```python
from build123d import *

# Parameters (mm, degrees)
SKETCH1_R               = 15
SKETCH1_R_2             = 1.55
BOSS_EXTRUDE1_DEPTH     = 2.8
BOSS_EXTRUDE2_START     = 2.8
SKETCH3_R               = 7.6
BOSS_EXTRUDE2_DEPTH     = 11
CUT_EXTRUDE1_DEPTH      = 26.306916051
CUT_EXTRUDE1_DEPTH_BACK = 26.306916051
SKETCH4_R               = 2.5
SKETCH5_R               = 5
CUT_EXTRUDE2_DEPTH      = 5.5
BOSS_EXTRUDE3_START     = 12
SKETCH7_R               = 7.6
SKETCH7_R_2             = 3.2
BOSS_EXTRUDE3_DEPTH     = 12
SKETCH8_R               = 3.2
SKETCH8_R_2             = 2.5
BOSS_EXTRUDE4_DEPTH     = 8
BOSS_EXTRUDE5_START     = 3
SKETCH9_R               = 8.25
SKETCH9_R_2             = 7.6
BOSS_EXTRUDE5_DEPTH     = 3
FILLET2_R               = 1
BOSS_EXTRUDE6_START     = 5.5
SKETCH11_R              = 5
SKETCH11_R_2            = 2.5
BOSS_EXTRUDE6_DEPTH     = 5.5
CUT_EXTRUDE3_DEPTH      = 5.5
BOSS_EXTRUDE7_START     = -18.3
SKETCH12_R              = 2.5
BOSS_EXTRUDE7_DEPTH     = 13.3


with BuildPart() as part:
    # Sketch1 → Boss-Extrude1 (new body)
    with BuildSketch(Plane.XY):
        Circle(SKETCH1_R)
        with Locations((0, 12.5)):
            Circle(SKETCH1_R_2, mode=Mode.SUBTRACT)
        with Locations((12.5, 0)):
            Circle(SKETCH1_R_2, mode=Mode.SUBTRACT)
        with Locations((0, -12.5)):
            Circle(SKETCH1_R_2, mode=Mode.SUBTRACT)
        with Locations((-12.5, 0)):
            Circle(SKETCH1_R_2, mode=Mode.SUBTRACT)
    extrude(amount=BOSS_EXTRUDE1_DEPTH)

    # Sketch3 → Boss-Extrude2 (add)
    with BuildSketch(Plane.XY.offset(BOSS_EXTRUDE2_START)):
        Circle(SKETCH3_R)
    extrude(amount=BOSS_EXTRUDE2_DEPTH)

    # Sketch4 → Cut-Extrude1 (cut, two sides: drawn at the far end of the back side and taken through both)
    with BuildSketch(Plane.XY.offset(13.8).offset(-CUT_EXTRUDE1_DEPTH_BACK)):
        Circle(SKETCH4_R)
    extrude(amount=CUT_EXTRUDE1_DEPTH + CUT_EXTRUDE1_DEPTH_BACK, mode=Mode.SUBTRACT)

    # Sketch5 → Cut-Extrude2 (cut)
    with BuildSketch(Plane.XY.offset(13.8)):
        Circle(SKETCH5_R)
    extrude(amount=-CUT_EXTRUDE2_DEPTH, mode=Mode.SUBTRACT)

    # Sketch7 → Boss-Extrude3 (add)
    with BuildSketch(Plane(origin=(0, 0, 0), x_dir=(-1, 0, 0), z_dir=(0, 0, -1)).offset(BOSS_EXTRUDE3_START)):
        with Locations(Location((0, 0, 0), (0, 0, 180))):
            Circle(SKETCH7_R)
        Circle(SKETCH7_R_2, mode=Mode.SUBTRACT)
    extrude(amount=-BOSS_EXTRUDE3_DEPTH)

    # Sketch8 → Boss-Extrude4 (add)
    with BuildSketch(Plane(origin=(0, 0, 0), x_dir=(-1, 0, 0), z_dir=(0, 0, -1))):
        Circle(SKETCH8_R)
        with Locations(Location((0, 0, 0), (0, 0, 180))):
            Circle(SKETCH8_R_2, mode=Mode.SUBTRACT)
    extrude(amount=BOSS_EXTRUDE4_DEPTH)

    # Sketch9 → Boss-Extrude5 (add)
    with BuildSketch(Plane(origin=(0, 0, 0), x_dir=(-1, 0, 0), z_dir=(0, 0, -1)).offset(BOSS_EXTRUDE5_START)):
        with Locations(Location((0, 0, 0), (0, 0, 180))):
            Circle(SKETCH9_R)
        with Locations(Location((0, 0, 0), (0, 0, 180))):
            Circle(SKETCH9_R_2, mode=Mode.SUBTRACT)
    extrude(amount=-BOSS_EXTRUDE5_DEPTH)

    # Fillet2
    fillet2_edges = [part.edges().sort_by_distance(p)[0] for p in [
        (-8.25, 0, 0),
    ]]
    fillet(fillet2_edges, radius=FILLET2_R)

    # Sketch11 → Boss-Extrude6 (add)
    with BuildSketch(Plane.XY.offset(8.3).offset(BOSS_EXTRUDE6_START)):
        Circle(SKETCH11_R)
        Circle(SKETCH11_R_2, mode=Mode.SUBTRACT)
    extrude(amount=-BOSS_EXTRUDE6_DEPTH)

    # Sketch10 → Cut-Extrude3 (cut)
    with BuildSketch(Plane.XY.offset(13.8)):
        with BuildLine():
            Line((0, 0), (5.412658774, -3.125))
            ThreePointArc((5.412658774, -3.125), (6.25, 0), (5.412658774, 3.125))
            Line((5.412658774, 3.125), (0, 0))
        make_face()
        with BuildLine():
            Line((-5.412658774, 3.125), (0, 0))
            Line((0, 0), (0, 6.25))
            ThreePointArc((0, 6.25), (-3.125, 5.412658774), (-5.412658774, 3.125))
        make_face()
        with BuildLine():
            Line((0, -6.25), (0, 0))
            Line((0, 0), (-5.412658774, -3.125))
            ThreePointArc((-5.412658774, -3.125), (-3.125, -5.412658774), (0, -6.25))
        make_face()
    extrude(amount=-CUT_EXTRUDE3_DEPTH, mode=Mode.SUBTRACT)

    # Sketch12 → Boss-Extrude7 (add)
    with BuildSketch(Plane(origin=(0, 0, -12), x_dir=(-1, 0, 0), z_dir=(0, 0, -1)).offset(BOSS_EXTRUDE7_START)):
        with Locations(Location((0, 0, 0), (0, 0, 180))):
            Circle(SKETCH12_R)
    extrude(amount=BOSS_EXTRUDE7_DEPTH)


solid = part.part
```
CAD build for the part. Positions are in the model's coordinates, mm. A direction names the side the tool comes from. Round coordinates to 2 decimals unless told otherwise and drop trailing zeros. Order: outer loops, then holes, each group sorted by start corner. A loop starts at its lowest first (then second) coordinate and runs counter-clockwise, first axis right, second up. Notation, with made-up numbers: (69.5, 0) - (106.5, 0) arc R25 cw to (106.5, 23) - close; hole circle Ø10 at (-27, -30.5). An arc over 180 degrees is marked (long way). Answer as CSV lines item,"result". Start each with the question number.
1. Saw through at B-B, the plane y = -12.5. Write the cut outline in (x, z), and give its area (3 significant figures).
2. Tool access for faces 4 (the face through (11.27, -0.94, 1.38)), 5 (the face through (2, -2, -8)), 6 (the face through (0, -4, 11)): list every direction of +Z, -Z, +X, -X, +Y, -Y with a clear straight run to the whole face (end or side of a thin tool).
3. Pull direction Y, two halves, no side cores. Call faces 1 (the face through (-14.985, 0.66, 1.38)), 2 (the face through (-3.81, 2.2, 11.09)), 3 (the face through (4, 7, -3)): +Y half, -Y half, draft (parallel to the pull), parting line (faces both ways), or undercut.
4. Saw through at C-C, the plane z = -8.5. Write the cut outline in (x, y), and give its area (3 significant figures).
5. Drill centre lines: L1, parallel to Y at x = 0, z = 0.75; L2, parallel to Z at x = -5, y = -8.5; L3, parallel to Y at x = -5, z = 9.75. Where is each one in solid material? Low to high. Write a range as [from, to].
6. Saw through at D-D, the plane z = -3.75. Write the cut outline in (x, y), and give its area (3 significant figures).
7. Saw through at A-A, the plane x = 13.25. Write the cut outline in (y, z).
8. Pin check, flat tips, straight feed: pin 1 (4 mm diameter, centred on y = -4.5, z = 12, fed in from -X); pin 2 (5 mm diameter, centred on y = -9.5, z = -5, fed in from -X); pin 3 (5 mm diameter, centred on x = 0, y = -12.5, fed in from -Z); pin 4 (1.9 mm diameter, centred on x = 0, y = 12.5, fed in from -Z). Stop position of each tip, or through.
Model answer:
1,outline,"(-8.29, 0) - (-1.55, 0) - (-1.55, 2.8) - (-8.29, 2.8) - close; (1.55, 0) - (8.29, 0) - (8.29, 2.8) - (1.55, 2.8) - close"
1,area,"37.8 mm²"
2,face 4,"+Z, -Z"
2,face 5,"-Z"
2,face 6,"+Z"
3,face 1,"parting line"
3,face 2,"undercut"
3,face 3,"draft"
4,outline,"circle Ø15.2 at (0, 0); hole circle Ø6.4 at (0, 0)"
4,area,"149 mm²"
5,L1,"y = [-15, -14.05], [-10.95, 10.95], [14.05, 15]"
5,L2,"z = [0, 2.8]"
5,L3,"y = [-5.72, -3.75], [-2.89, 2.89], [3.75, 5.72]"
6,outline,"circle Ø15.2 at (0, 0)"
6,area,"181 mm²"
7,outline,"(-7.03, 0) - (-1.36, 0) - (-1.36, 2.8) - (-7.03, 2.8) - close; (1.36, 0) - (7.03, 0) - (7.03, 2.8) - (1.36, 2.8) - close"
8,pin 1,"stops at x = -7.18"
8,pin 2,"stops at x = -2.96"
8,pin 3,"stops at z = 0"
8,pin 4,"passes through"
